Check sheet for the modelled part. Datum: model origin and axes. Units: mm. Give positions to 0.01 mm unless a question says otherwise; leave off trailing zeros. Write each loop counter-clockwise with the first axis right and the second up, starting at its lowest first coordinate (ties: lowest second). Pieces come first, ordered by that corner, then holes. Notation, with made-up numbers: (-27, 32) -> (2, 32) arc R14 cw to (2, 46) -> close; hole circle Ø2 at (79, 54). An arc over 180 degrees is marked (long way). Return JSON: item names as keys, results as strings.
from build123d import *

# Parameters (mm, degrees)
CYLINDER010_R     = 1.55
CYLINDER010_DEPTH = 10
CYLINDER011_R     = 1.55
CYLINDER011_DEPTH = 10
CYLINDER012_R     = 1.55
CYLINDER012_DEPTH = 10
CYLINDER_R        = 1.55
CYLINDER_DEPTH    = 10
BOX_W             = 56.21
BOX_H             = 65.15
BOX_DEPTH         = 10
FILLET024_R       = 2


with BuildPart() as cylinder010:
    # Cylinder010 → Cylinder010 (new body)
    with BuildSketch(Plane(origin=(3.5, 61.52, 0), x_dir=(1, 0, 0), z_dir=(0, 0, 1))):
        Circle(CYLINDER010_R)
    extrude(amount=CYLINDER010_DEPTH)


with BuildPart() as cylinder011:
    # Cylinder011 → Cylinder011 (new body)
    with BuildSketch(Plane(origin=(52.71, 3.5, 0), x_dir=(1, 0, 0), z_dir=(0, 0, 1))):
        Circle(CYLINDER011_R)
    extrude(amount=CYLINDER011_DEPTH)


with BuildPart() as cylinder012:
    # Cylinder012 → Cylinder012 (new body)
    with BuildSketch(Plane(origin=(52.71, 61.52, 0), x_dir=(1, 0, 0), z_dir=(0, 0, 1))):
        Circle(CYLINDER012_R)
    extrude(amount=CYLINDER012_DEPTH)


with BuildPart() as fusion_holes:
    # Cylinder → Cylinder (new body)
    with BuildSketch(Plane(origin=(3.5, 3.5, 0), x_dir=(1, 0, 0), z_dir=(0, 0, 1))):
        Circle(CYLINDER_R)
    extrude(amount=CYLINDER_DEPTH)

    # Fusion: union Cylinder010, Cylinder011, Cylinder012
    add(cylinder010.part)
    add(cylinder011.part)
    add(cylinder012.part)


with BuildPart() as board:
    # Box → Box (new body)
    with BuildSketch(Plane.XY):
        with Locations((28.105, 32.575)):
            Rectangle(BOX_W, BOX_H)
    extrude(amount=BOX_DEPTH)

    # Fillet024
    fillet024_edges = [board.edges().sort_by_distance(p)[0] for p in [
        (0, 0, 5),
        (0, 65.15, 5),
        (56.21, 0, 5),
        (56.21, 65.15, 5),
    ]]
    fillet(fillet024_edges, radius=FILLET024_R)

    # Cut: cut Fusion - holes
    add(fusion_holes.part, mode=Mode.SUBTRACT)


with BuildPart() as board_1:
    # Cut placement: moved
    add(board.part.moved(Location((0, 2.5, 19))))


solid = board_1.part
(1) Cross-section at A-A on y = 64.02. Enter the section's corners in (x, z).
Reply:
{"outline": "(0, 19) -> (1.95, 19) -> (1.95, 29) -> (0, 29) -> close; (5.05, 19) -> (51.16, 19) -> (51.16, 29) -> (5.05, 29) -> close; (54.26, 19) -> (56.21, 19) -> (56.21, 29) -> (54.26, 29) -> close"}
(2) Depth check by flat-ended pin: pin 1 Ø1.9 at (x, y) = (3.5, 6) entering from -Z. Enter the tip coordinate at first touch or a pass-through.
Reply:
{"pin 1": "through"}
(3) Cross-section at B-B on x = 3.5. Enter the section's corners in (y, z).
Reply:
{"outline": "(2.5, 19) -> (4.45, 19) -> (4.45, 29) -> (2.5, 29) -> close; (7.55, 19) -> (62.47, 19) -> (62.47, 29) -> (7.55, 29) -> close; (65.57, 19) -> (67.65, 19) -> (67.65, 29) -> (65.57, 29) -> close"}
(4) Thickness scan on L1, parallel to Y at x = 3.5, z = 22.75; L2, parallel to Y at x = 53, z = 22.25; L3, parallel to X at y = 5, z = 21.5. Record the ranges inside material, lowest first.
Reply:
{"L1": "2.5 to 4.45, 7.55 to 62.47, 65.57 to 67.65", "L2": "2.5 to 4.48, 7.52 to 62.5, 65.54 to 67.65", "L3": "0 to 2.32, 4.68 to 51.53, 53.89 to 56.21"}
(5) Release check for a two-part mould opening along X. For faces 1 (the cylindrical face through (2.36, 7.05, 23.93)), 2 (the flat face through (28, 36, 29)), 3 (the cylindrical face through (55.61, 3.07, 24.07)), 4 (the cylindrical face through (54.188, 6.466, 23.93)) record: pulls with the +X half, pulls with the -X half, needs draft (parallel to the pull), parting line crosses it, or undercut.
Reply:
{"face 1": "undercut", "face 2": "needs draft", "face 3": "pulls with the +X half", "face 4": "undercut"}
